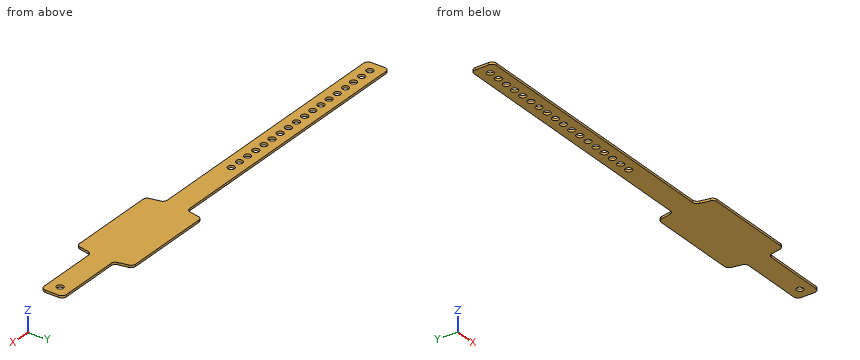
from build123d import *

# Parameters (mm, degrees)
BOSS_EXTRUDE1_DEPTH = 1
BOSS_EXTRUDE2_DEPTH = 1
FILLET1_R           = 2
SKETCH4_R           = 1.5
CUT_EXTRUDE1_DEPTH  = 201.766655598


with BuildPart() as part:
    # Sketch2 → Boss-Extrude1 (new body)
    with BuildSketch(Plane.XY):
        with BuildLine():
            Line((2, 0), (198, 0))
            ThreePointArc((198, 0), (199.414213562, 0.585786438), (200, 2))
            Line((200, 2), (200, 8))
            ThreePointArc((200, 8), (199.414213562, 9.414213562), (198, 10))
            Line((198, 10), (2, 10))
            ThreePointArc((2, 10), (0.585786438, 9.414213562), (0, 8))
            Line((0, 8), (0, 2))
            ThreePointArc((0, 2), (0.585786438, 0.585786438), (2, 0))
        make_face()
    extrude(amount=BOSS_EXTRUDE1_DEPTH)

    # Sketch3 → Boss-Extrude2 (add)
    with BuildSketch(Plane(origin=(0, 0, 0), x_dir=(-1, 0, 0), z_dir=(0, 0, -1))):
        with BuildLine():
            Line((-124, 0), (-125.178446454, -5.89223227))
            ThreePointArc((-125.178446454, -5.89223227), (-125.871629994, -7.046684283), (-127.139607805, -7.5))
            Line((-127.139607805, -7.5), (-165.860392195, -7.5))
            ThreePointArc((-165.860392195, -7.5), (-167.128370006, -7.046684283), (-167.821553546, -5.89223227))
            Line((-167.821553546, -5.89223227), (-169, 0))
            Line((-169, 0), (-124, 0))
        make_face()
        with BuildLine():
            Line((-169, 10), (-124, 10))
            Line((-124, 10), (-125.178446454, 15.89223227))
            ThreePointArc((-125.178446454, 15.89223227), (-125.871629994, 17.046684283), (-127.139607805, 17.5))
            Line((-127.139607805, 17.5), (-165.860392195, 17.5))
            ThreePointArc((-165.860392195, 17.5), (-167.128370006, 17.046684283), (-167.821553546, 15.89223227))
            Line((-167.821553546, 15.89223227), (-169, 10))
        make_face()
    extrude(amount=-BOSS_EXTRUDE2_DEPTH)

    # Fillet1
    fillet1_edges = [part.edges().sort_by_distance(p)[0] for p in [
        (169, 0, 0.5),
        (124, 0, 0.5),
        (124, 10, 0.5),
        (169, 10, 0.5),
    ]]
    fillet(fillet1_edges, radius=FILLET1_R)

    # Sketch4 → Cut-Extrude1 (cut, through all)
    with BuildSketch(Plane(origin=(0, 0, 0), x_dir=(-1, 0, 0), z_dir=(0, 0, -1))):
        with Locations((-5, 5)):
            Circle(SKETCH4_R)
        with Locations((-10, 5)):
            Circle(SKETCH4_R)
        with Locations((-15, 5)):
            Circle(SKETCH4_R)
        with Locations((-20, 5)):
            Circle(SKETCH4_R)
        with Locations((-25, 5)):
            Circle(SKETCH4_R)
        with Locations((-30, 5)):
            Circle(SKETCH4_R)
        with Locations((-195, 5)):
            Circle(SKETCH4_R)
        with Locations((-35, 5)):
            Circle(SKETCH4_R)
        with Locations((-40, 5)):
            Circle(SKETCH4_R)
        with Locations((-45, 5)):
            Circle(SKETCH4_R)
        with Locations((-50, 5)):
            Circle(SKETCH4_R)
        with Locations((-55, 5)):
            Circle(SKETCH4_R)
        with Locations((-60, 5)):
            Circle(SKETCH4_R)
        with Locations((-65, 5)):
            Circle(SKETCH4_R)
        with Locations((-70, 5)):
            Circle(SKETCH4_R)
        with Locations((-75, 5)):
            Circle(SKETCH4_R)
        with Locations((-80, 5)):
            Circle(SKETCH4_R)
        with Locations((-85, 5)):
            Circle(SKETCH4_R)
        with Locations((-90, 5)):
            Circle(SKETCH4_R)
    extrude(amount=-CUT_EXTRUDE1_DEPTH, mode=Mode.SUBTRACT)


solid = part.part
Input: part model. Units: mm. Frame: model coordinates. Round coordinates to 2 decimals unless told otherwise and drop trailing zeros. Write each loop counter-clockwise with the first axis right and the second up, starting at its lowest first coordinate (ties: lowest second). Pieces come first, ordered by that corner, then holes.
1) Cut plane A-A (z = 0.7). Count the separate pieces of the cut face and the enclosed holes in it, then the cut area to 3 significant figures.
2) Ray query, L1, parallel to Y at x = 65, z = 0.7; L2, parallel to X at y = 1.75, z = 0.75; L3, parallel to Y at x = 180.5, z = 0.85. Return the intervals inside material, ascending.
3) Cut plane C-C (y = 13.75). Return the cut outline in (x, z), then the cut area to 3 significant figures.
4) Cut plane B-B (x = 112). Return the cut outline in (y, z).
5) Contact query for flat-ended pins moving along their axis: P1, Ø2.5, axis at x = 85, y = 5, coming from the -Z side; P2, Ø3.5, axis at x = 75, y = 5, coming from the -Z side. Output: stop coordinate, or through.
Geometry says:
1. separate pieces: 1
1. enclosed holes: 19
1. area: 2,510 mm2
2. L1: y = 0 to 3.5, 6.5 to 10
2. L2: x = 0.02 to 199.98
2. L3: y = 0 to 10
3. outline: (124.75, 0) - (168.25, 0) - (168.25, 1) - (124.75, 1) - close
3. area: 43.5 mm2
4. outline: (0, 0) - (10, 0) - (10, 1) - (0, 1) - close
5. P1: passes through
5. P2: stops at z = 0
